Design review of the part built by this model. Coordinates are the model's own, in mm. A direction names the side the tool comes from. Give positions to 0.01 mm unless a question says otherwise; leave off trailing zeros. Loops run counter-clockwise (first coordinate to the right, second up) from the corner with the lowest first, then second, coordinate; pieces in that order, holes last.
from build123d import *

# Parameters (mm, degrees)
SKETCH1_W           = 40
SKETCH1_H           = 20
BOSS_EXTRUDE1_DEPTH = 40
CUT_EXTRUDE18_DEPTH = 20
CUT_EXTRUDE20_DEPTH = 59
CUT_EXTRUDE21_DEPTH = 59
SKETCH13_W          = 56.232322264
SKETCH13_H          = 131.72647096
CUT_EXTRUDE22_DEPTH = 20
REVOLVE1_ANGLE      = 180
CUT_EXTRUDE23_DEPTH = 20


with BuildPart() as part:
    # Sketch1 → Boss-Extrude1 (new body)
    with BuildSketch(Plane.XY):
        with BuildLine():
            Line((0, 20), (40, 20))
            ThreePointArc((40, 20), (20, 40), (0, 20))
        make_face()
        with Locations((20, 10)):
            Rectangle(SKETCH1_W, SKETCH1_H)
    extrude(amount=BOSS_EXTRUDE1_DEPTH)

    # Sketch4 → Cut-Extrude18 (cut)
    with BuildSketch(Plane.XY.offset(40)):
        with BuildLine():
            Line((20, 30), (20, 20))
            Line((20, 20), (10, 20))
            ThreePointArc((10, 20), (12.928932188, 27.071067812), (20, 30))
        make_face()
    extrude(amount=-CUT_EXTRUDE18_DEPTH, mode=Mode.SUBTRACT)

    # Sketch11 → Cut-Extrude20 (cut)
    with BuildSketch(Plane(origin=(0, 0, 0), x_dir=(1, 0, 0), z_dir=(0, 1, 0))):
        Polygon((20, -40), (0, 0), (0, -40), align=None)
        Polygon((40, 0), (20, -40), (40, -40), align=None)
    extrude(amount=CUT_EXTRUDE20_DEPTH, mode=Mode.SUBTRACT)

    # Sketch12 → Cut-Extrude21 (cut)
    with BuildSketch(Plane(origin=(0, 0, 0), x_dir=(0, 0, -1), z_dir=(1, 0, 0))):
        Polygon((-40, 20), (0, 40), (-40, 40), align=None)
    extrude(amount=CUT_EXTRUDE21_DEPTH, mode=Mode.SUBTRACT)

    # Sketch13 → Cut-Extrude22 (cut)
    with BuildSketch(Plane(origin=(0, 20, 0), x_dir=(1, 0, 0), z_dir=(0, 1, 0))):
        with Locations((25.992745576, -5.369768382)):
            Rectangle(SKETCH13_W, SKETCH13_H)
    extrude(amount=CUT_EXTRUDE22_DEPTH, mode=Mode.SUBTRACT)

    # Sketch14 → Revolve1 (revolve)
    with BuildSketch(Plane(origin=(0, 20, 0), x_dir=(1, 0, 0), z_dir=(0, 1, 0))):
        Polygon((20, -40), (20, 0), (0, 0), align=None)
    revolve(axis=Axis((20, 20, 40), (0, 0, -1)), revolution_arc=REVOLVE1_ANGLE)

    # Sketch15 → Cut-Extrude23 (cut)
    with BuildSketch(Plane(origin=(0, 20, 0), x_dir=(1, 0, 0), z_dir=(0, 1, 0))):
        Polygon((20, -40), (20, -20), (10, -20), align=None)
    extrude(amount=CUT_EXTRUDE23_DEPTH, mode=Mode.SUBTRACT)


solid = part.part
Q1. Insertion check: pin 1 (6 mm diameter, centred on y = 22, z = 30, fed in from +X); pin 2 (3 mm diameter, centred on x = 34, z = 15.5, fed in from -Y); pin 3 (11 mm diameter, centred on y = 22.5, z = 30, fed in from -X); pin 4 (8 mm diameter, centred on y = 5.5, z = 6, fed in from -X). Each pin has a flat end and moves straight along its axis. Give the tip position at first contact, or say it passes through.
Results:
pin 1: stops at x = 26.34
pin 2: passes through
pin 3: stops at x = 12.55
pin 4: stops at x = 1
Q2. Take a section at D-D (z = 7). Give the boundary of the cut face in (x, y), plus the area to 3 significant figures.
Results:
outline: (3.5, 0) - (36.5, 0) - (36.5, 20) arc R16.5 ccw to (3.5, 20) - close
area: 1,090 mm2
Q3. Tool access review of faces 1 (the face through (20, 20, 0)), 2 (the face through (20, 23, 26)): name each direction out of +Z, -Z, +X, -X, +Y, -Y from which nothing blocks a thin tool from reaching the whole face with its end or side.
Results:
face 1: -Z, +X, -X, +Y, -Y
face 2: +Z, -X, +Y
Q4. Take a section at C-C (z = 35). Give the boundary of the cut face in (x, y), plus the area to 3 significant figures.
Results:
outline: (17.5, 0) - (22.5, 0) - (22.5, 20) arc R2.5 ccw to (20, 22.5) - (20, 20) - (17.5, 20) - close
area: 105 mm2
Q5. Take a section at A-A (z = 27). Give the boundary of the cut face in (x, y), plus the area to 3 significant figures.
Results:
outline: (13.5, 0) - (26.5, 0) - (26.5, 20) arc R6.5 ccw to (20, 26.5) - (20, 20) - (13.5, 20) - close
area: 293 mm2
Q6. Wall thickness on line 1 (Z direction, x = 15, y = 7.5); line 2 (Z direction, x = 15, y = 22.5); line 3 (X direction, y = 2, z = 2): over which ranges is each line inside the solid? List them lowest first.
Results:
line 1: z = 0 to 30
line 2: z = 0 to 20
line 3: x = 1 to 39
Q7. Take a section at B-B (y = 10). Give the boundary of the cut face in (x, z), plus the area to 3 significant figures.
Results:
outline: (0, 0) - (40, 0) - (20, 40) - close
area: 800 mm2
